For this review, take the finished solid that the model builds, in its own axes (mm). Coordinates: 2 decimals unless noted, no trailing zeros. Write each loop counter-clockwise with the first axis right and the second up, starting at its lowest first coordinate (ties: lowest second). Pieces come first, ordered by that corner, then holes. Notation, with made-up numbers: (74, 59.5) -> (86, 59.5) arc R16 cw to (86, 66.5) -> close; hole circle Ø2 at (56.5, -8). An arc over 180 degrees is marked (long way). Put each result on its own line as item: value. Start each with the question number.
Item 1: Consider section A-A on z = 9.5. Give the boundary of the cut face in (x, y), and give its area (3 significant figures).
Item 2: The part is to be moulded in two halves that separate along Y. For faces 1 (the cylindrical face through (88.46, -8.56, 2.85)), 2 (the flat face through (88, 22, 71)), 3 (the flat face through (88, 0, 149)), say which applies: +Y half, -Y half, draft (parallel to the pull), parting line (faces both ways), or undercut.
Item 3: Insertion check: P1, Ø3, axis at y = 12, z = 141.5, coming from the +X side. The pin has a flat end and moves straight along its axis. Give the tip position at first contact, or say it passes through.
Item 4: Consider section B-B on y = -7. Give the boundary of the cut face in (x, z).
Item 5: To check wall thickness, follow L1, parallel to Z at x = 88.45, y = 12; L2, parallel to Z at x = 88.3, y = -7; L3, parallel to Y at x = 89.75, z = 141.5. State the ranges of each line that lie inside material, in increasing order.
```python
from build123d import *

# Parameters (mm, degrees)
CYLINDER019_R           = 1.6
CYLINDER019_DEPTH       = 40
CYLINDER019_PITCH_ANGLE = 90
CYLINDER018_R           = 1.6
CYLINDER018_DEPTH       = 40
CYLINDER018_PITCH_ANGLE = 90
CYLINDER017_R           = 1.6
CYLINDER017_DEPTH       = 40
CYLINDER016_R           = 1.6
CYLINDER016_DEPTH       = 70
CYLINDER016_ROLL_ANGLE  = 90
CYLINDER015_R           = 1.6
CYLINDER015_DEPTH       = 40
BOX015_W                = 5
BOX015_H                = 45
BOX015_DEPTH            = 154


with BuildPart() as cylinder100:
    # Cylinder019 → Cylinder019 (new body)
    with BuildSketch(Plane.XY):
        Circle(CYLINDER019_R)
    extrude(amount=CYLINDER019_DEPTH)


with BuildPart() as cylinder100_1:
    # Cylinder019 pitch: moved
    add(cylinder100.part.rotate(Axis((0, 0, 0), (0, 1, 0)), CYLINDER019_PITCH_ANGLE))


with BuildPart() as cylinder100_2:
    # Cylinder019 placement: moved
    add(cylinder100_1.part.moved(Location((-40, 12, 9.5))))


with BuildPart() as fusion011:
    # Cylinder018 → Cylinder018 (new body)
    with BuildSketch(Plane.XY):
        Circle(CYLINDER018_R)
    extrude(amount=CYLINDER018_DEPTH)


with BuildPart() as fusion011_1:
    # Cylinder018 pitch: moved
    add(fusion011.part.rotate(Axis((0, 0, 0), (0, 1, 0)), CYLINDER018_PITCH_ANGLE))


with BuildPart() as fusion011_2:
    # Cylinder018 placement: moved
    add(fusion011_1.part.moved(Location((-40, -7, 2.5))))

    # Fusion011: union Cylinder100
    add(cylinder100_2.part)


with BuildPart() as fusion012:
    # Cylinder017 → Cylinder017 (new body)
    with BuildSketch(Plane(origin=(-27.5, 7, -15), x_dir=(1, 0, 0), z_dir=(0, 0, 1))):
        Circle(CYLINDER017_R)
    extrude(amount=CYLINDER017_DEPTH)

    # Fusion012: union Fusion011
    add(fusion011_2.part)


with BuildPart() as fusion013:
    # Cylinder016 → Cylinder016 (new body)
    with BuildSketch(Plane.XY):
        Circle(CYLINDER016_R)
    extrude(amount=CYLINDER016_DEPTH)


with BuildPart() as fusion013_1:
    # Cylinder016 roll: moved
    add(fusion013.part.rotate(Axis((0, 0, 0), (1, 0, 0)), CYLINDER016_ROLL_ANGLE))


with BuildPart() as fusion013_2:
    # Cylinder016 placement: moved
    add(fusion013_1.part.moved(Location((-24, 39, 6))))

    # Fusion013: union Fusion012
    add(fusion012.part)


with BuildPart() as cylinder008:
    # Cylinder015 → Cylinder015 (new body)
    with BuildSketch(Plane(origin=(-20.5, -12, -15), x_dir=(1, 0, 0), z_dir=(0, 0, 1))):
        Circle(CYLINDER015_R)
    extrude(amount=CYLINDER015_DEPTH)


with BuildPart() as face_corner_holes013:
    # Fusion027 base: copy of Cylinder008
    add(cylinder008.part)

    # Fusion027: union Fusion013
    add(fusion013_2.part)


with BuildPart() as face_corner_holes013_1:
    # Fusion027 placement: moved
    add(face_corner_holes013.part.moved(Location((104, 0, 132))))


with BuildPart() as face_corner_holes001:
    # Fusion015 base: copy of Cylinder008
    add(cylinder008.part)

    # Fusion015: union Fusion013
    add(fusion013_2.part)


with BuildPart() as face_corner_holes001_1:
    # Fusion015 placement: moved
    add(face_corner_holes001.part.moved(Location((104, 0, 0))))


with BuildPart() as top_x:
    # Box015 → Box015 (new body)
    with BuildSketch(Plane(origin=(86, -23, -5), x_dir=(1, 0, 0), z_dir=(0, 0, 1))):
        with Locations((2.5, 22.5)):
            Rectangle(BOX015_W, BOX015_H)
    extrude(amount=BOX015_DEPTH)

    # Cut016: cut face-corner-holes001
    add(face_corner_holes001_1.part, mode=Mode.SUBTRACT)

    # Cut024: cut face-corner-holes013
    add(face_corner_holes013_1.part, mode=Mode.SUBTRACT)


solid = top_x.part
```
Return value:
1. outline: (86, -23) -> (91, -23) -> (91, 10.4) -> (86, 10.4) -> close; (86, 13.6) -> (91, 13.6) -> (91, 22) -> (86, 22) -> close
1. area: 209 mm^2
2. face 1: undercut
2. face 2: +Y half
2. face 3: draft
3. P1: through
4. outline: (86, -5) -> (91, -5) -> (91, 0.9) -> (86, 0.9) -> close; (86, 4.1) -> (91, 4.1) -> (91, 132.9) -> (86, 132.9) -> close; (86, 136.1) -> (91, 136.1) -> (91, 149) -> (86, 149) -> close
5. L1: -5 to 7.9, 11.1 to 139.9, 143.1 to 149
5. L2: -5 to 0.9, 4.1 to 132.9, 136.1 to 149
5. L3: -23 to 10.4, 13.6 to 22
